```python
from build123d import *

# Parameters (mm, degrees)
SKETCH1_W                                            = 550
SKETCH1_H                                            = 360
BOSS_EXTRUDE1_DEPTH                                  = 5
SKETCH2_W                                            = 40
SKETCH2_H                                            = 15
CUT_EXTRUDE1_DEPTH                                   = 10
FILLET1_R                                            = 7.5
CHAMFER1_SIZE                                        = 50
SKETCH8_R                                            = 1.5
CUT_EXTRUDE5_DEPTH                                   = 10
CSK_FOR_M4_HEX_SOCKET_COUNTERSUNK_HEAD_S_D           = 4.5
CSK_FOR_M4_HEX_SOCKET_COUNTERSUNK_HEAD_S_CSINK_D     = 9.18
CSK_FOR_M4_HEX_SOCKET_COUNTERSUNK_HEAD_S_CSINK_ANGLE = 90
SKETCH10_R                                           = 2
CUT_EXTRUDE6_DEPTH                                   = 10
M5_TAPPED_HOLE1_D                                    = 4.2
M5_TAPPED_HOLE1_DEPTH                                = 12.4
M5_TAPPED_HOLE1_TIP                                  = 1.2618073
CUT_EXTRUDE8_REACH                                   = 330.71
SKETCH14_R                                           = 1.25
M3_TAPPED_HOLE1_D                                    = 2.5
M3_TAPPED_HOLE1_DEPTH                                = 7.5
M3_TAPPED_HOLE1_TIP                                  = 0.751075774
SKETCH16_R                                           = 1.5
CUT_EXTRUDE9_DEPTH                                   = 329.709598278
CSK_FOR_M4_HEX_SOCKET_COUNTERSUNK_HE_2_D             = 4.5
CSK_FOR_M4_HEX_SOCKET_COUNTERSUNK_HE_2_CSINK_D       = 9.18
CSK_FOR_M4_HEX_SOCKET_COUNTERSUNK_HE_2_CSINK_ANGLE   = 90


with BuildPart() as part:
    # Sketch1 → Boss-Extrude1 (new body)
    with BuildSketch(Plane(origin=(0, 0, 0), x_dir=(1, 0, 0), z_dir=(0, 1, 0))):
        Rectangle(SKETCH1_W, SKETCH1_H)
    extrude(amount=BOSS_EXTRUDE1_DEPTH)

    # Sketch2 → Cut-Extrude1 (cut)
    with BuildSketch(Plane(origin=(0, 5, 0), x_dir=(1, 0, 0), z_dir=(0, 1, 0))):
        with Locations((195, 0)):
            Rectangle(SKETCH2_W, SKETCH2_H)
        with Locations((-195, 0)):
            Rectangle(SKETCH2_W, SKETCH2_H)
    extrude(amount=-CUT_EXTRUDE1_DEPTH, mode=Mode.SUBTRACT)

    # Fillet1
    fillet1_edges = [part.edges().sort_by_distance(p)[0] for p in [
        (-175, 2.5, 7.5),
        (-175, 2.5, -7.5),
        (-215, 2.5, -7.5),
        (-215, 2.5, 7.5),
        (175, 2.5, 7.5),
        (175, 2.5, -7.5),
        (215, 2.5, -7.5),
        (215, 2.5, 7.5),
    ]]
    fillet(fillet1_edges, radius=FILLET1_R - 0.0001)  # a hair under: the kernel refuses the full size

    # Chamfer1
    chamfer1_edges = [part.edges().sort_by_distance(p)[0] for p in [
        (275, 2.5, 180),
        (-275, 2.5, 180),
        (-275, 2.5, -180),
        (275, 2.5, -180),
    ]]
    chamfer(chamfer1_edges, length=CHAMFER1_SIZE)

    # Sketch8 → Cut-Extrude5 (cut)
    with BuildSketch(Plane(origin=(0, 5, 0), x_dir=(1, 0, 0), z_dir=(0, 1, 0))):
        with Locations(Location((225, 5, 0), (0, 0, 270))):
            Circle(SKETCH8_R)
        with Locations(Location((165, 5, 0), (0, 0, 90))):
            Circle(SKETCH8_R)
        with Locations(Location((165, -5, 0), (0, 0, 270))):
            Circle(SKETCH8_R)
        with Locations(Location((225, -5, 0), (0, 0, 90))):
            Circle(SKETCH8_R)
        with Locations(Location((-225, -5, 0), (0, 0, 270))):
            Circle(SKETCH8_R)
        with Locations(Location((-165, -5, 0), (0, 0, 90))):
            Circle(SKETCH8_R)
        with Locations(Location((-165, 5, 0), (0, 0, 270))):
            Circle(SKETCH8_R)
        with Locations(Location((-225, 5, 0), (0, 0, 90))):
            Circle(SKETCH8_R)
    extrude(amount=-CUT_EXTRUDE5_DEPTH, mode=Mode.SUBTRACT)

    # CSK for M4 Hex Socket Countersunk Head S (through all)
    with Locations(Plane(origin=(-225, 5, -5), x_dir=(0, 0, 1), z_dir=(0, 1, 0))):
        with Locations((0, 0), (10, 0), (10, 60), (0, 60), (10, 390), (0, 390), (0, 450), (10, 450)):
            CounterSinkHole(CSK_FOR_M4_HEX_SOCKET_COUNTERSUNK_HEAD_S_D / 2, CSK_FOR_M4_HEX_SOCKET_COUNTERSUNK_HEAD_S_CSINK_D / 2, counter_sink_angle=CSK_FOR_M4_HEX_SOCKET_COUNTERSUNK_HEAD_S_CSINK_ANGLE)

    # Sketch10 → Cut-Extrude6 (cut)
    with BuildSketch(Plane(origin=(0, 5, 0), x_dir=(1, 0, 0), z_dir=(0, 1, 0))):
        with Locations(Location((237.5, 112, 0), (0, 0, 270))):
            Circle(SKETCH10_R)
        with Locations(Location((162.5, 112, 0), (0, 0, 90))):
            Circle(SKETCH10_R)
    extrude(amount=-CUT_EXTRUDE6_DEPTH, mode=Mode.SUBTRACT)

    # M5 Tapped Hole1
    with Locations(Plane(origin=(237.5, 5, -112), x_dir=(0, 0, 1), z_dir=(0, 1, 0))):
        with Locations((0, 0), (0, -75)):
            Hole(M5_TAPPED_HOLE1_D / 2, depth=M5_TAPPED_HOLE1_DEPTH)
            with Locations((0, 0, -(M5_TAPPED_HOLE1_DEPTH + M5_TAPPED_HOLE1_TIP / 2))):  # 118° drill point
                Cone(0, M5_TAPPED_HOLE1_D / 2, M5_TAPPED_HOLE1_TIP, mode=Mode.SUBTRACT)

    # Sketch14 → Cut-Extrude8 (cut, up to next)
    with BuildSketch(Plane(origin=(0, 5, 0), x_dir=(-1, 0, 0), z_dir=(0, 1, 0)), mode=Mode.PRIVATE) as cut_extrude8_sk1:
        with Locations(Location((-225, 25, 0), (0, 0, 90))):
            Circle(SKETCH14_R)
    cut_extrude8_tool1 = extrude(cut_extrude8_sk1.sketch, amount=-CUT_EXTRUDE8_REACH, mode=Mode.PRIVATE) & part.part
    # Sketch14 → Cut-Extrude8 (cut, up to next)
    with BuildSketch(Plane(origin=(0, 5, 0), x_dir=(-1, 0, 0), z_dir=(0, 1, 0)), mode=Mode.PRIVATE) as cut_extrude8_sk2:
        with Locations(Location((-225, -25, 0), (0, 0, 270))):
            Circle(SKETCH14_R)
    cut_extrude8_tool2 = extrude(cut_extrude8_sk2.sketch, amount=-CUT_EXTRUDE8_REACH, mode=Mode.PRIVATE) & part.part
    # Sketch14 → Cut-Extrude8 (cut, up to next)
    with BuildSketch(Plane(origin=(0, 5, 0), x_dir=(-1, 0, 0), z_dir=(0, 1, 0)), mode=Mode.PRIVATE) as cut_extrude8_sk3:
        with Locations(Location((-165, 25, 0), (0, 0, 270))):
            Circle(SKETCH14_R)
    cut_extrude8_tool3 = extrude(cut_extrude8_sk3.sketch, amount=-CUT_EXTRUDE8_REACH, mode=Mode.PRIVATE) & part.part
    # Sketch14 → Cut-Extrude8 (cut, up to next)
    with BuildSketch(Plane(origin=(0, 5, 0), x_dir=(-1, 0, 0), z_dir=(0, 1, 0)), mode=Mode.PRIVATE) as cut_extrude8_sk4:
        with Locations(Location((-165, -25, 0), (0, 0, 90))):
            Circle(SKETCH14_R)
    cut_extrude8_tool4 = extrude(cut_extrude8_sk4.sketch, amount=-CUT_EXTRUDE8_REACH, mode=Mode.PRIVATE) & part.part
    add(cut_extrude8_tool1.solids().sort_by_distance((225, 5, 25))[0], mode=Mode.SUBTRACT)
    add(cut_extrude8_tool2.solids().sort_by_distance((225, 5, -25))[0], mode=Mode.SUBTRACT)
    add(cut_extrude8_tool3.solids().sort_by_distance((165, 5, 25))[0], mode=Mode.SUBTRACT)
    add(cut_extrude8_tool4.solids().sort_by_distance((165, 5, -25))[0], mode=Mode.SUBTRACT)

    # M3 Tapped Hole1
    with Locations(Plane(origin=(225, 5, 25), x_dir=(0, 0, 1), z_dir=(0, 1, 0))):
        with Locations((0, 0), (0, -60), (-50, -60), (-50, 0)):
            Hole(M3_TAPPED_HOLE1_D / 2, depth=M3_TAPPED_HOLE1_DEPTH)
            with Locations((0, 0, -(M3_TAPPED_HOLE1_DEPTH + M3_TAPPED_HOLE1_TIP / 2))):  # 118° drill point
                Cone(0, M3_TAPPED_HOLE1_D / 2, M3_TAPPED_HOLE1_TIP, mode=Mode.SUBTRACT)

    # Sketch16 → Cut-Extrude9 (cut, through all)
    with BuildSketch(Plane(origin=(0, 5, 0), x_dir=(1, 0, 0), z_dir=(0, 1, 0))):
        with Locations(Location((38.6, 10.7, 0), (0, 0, 270))):
            Circle(SKETCH16_R)
        with Locations(Location((60, 10.7, 0), (0, 0, 270))):
            Circle(SKETCH16_R)
        with Locations(Location((38.6, -10.7, 0), (0, 0, 270))):
            Circle(SKETCH16_R)
        with Locations(Location((60, -10.7, 0), (0, 0, 270))):
            Circle(SKETCH16_R)
    extrude(amount=-CUT_EXTRUDE9_DEPTH, mode=Mode.SUBTRACT)

    # CSK for M4 Hex Socket Countersunk He 2 (through all)
    with Locations(Plane(origin=(60, 0, -10.7), x_dir=(0, 0, -1), z_dir=(0, -1, 0))):
        with Locations((0, 0), (0, -21.4), (-21.4, -21.4), (-21.4, 0)):
            CounterSinkHole(CSK_FOR_M4_HEX_SOCKET_COUNTERSUNK_HE_2_D / 2, CSK_FOR_M4_HEX_SOCKET_COUNTERSUNK_HE_2_CSINK_D / 2, counter_sink_angle=CSK_FOR_M4_HEX_SOCKET_COUNTERSUNK_HE_2_CSINK_ANGLE)


solid = part.part
```
Model file for the job. Use its own axes, mm. Coordinates: 2 decimals unless noted, no trailing zeros. Return JSON: item names as keys, results as strings. Group by question number.
1) Saw through at A-A, the plane y = 1.3. Count the separate pieces of the cut face and the enclosed holes in it, plus the area to 3 significant figures.
2) Flat gauge pins, fed straight in: P1, Ø2.5, axis at x = -225, z = -5, coming from the +Y side; P2, Ø7, axis at x = -225, z = 5, coming from the +Y side; P3, Ø5, axis at x = 38.6, z = -10.7, coming from the -Y side. Where does each tip first touch, or does it go through?
3) Probe line 1 (Z direction, x = 165, y = 1.9); line 2 (X direction, y = 1.6, z = 25); line 3 (Z direction, x = 39, y = 2.65). List the from-to ranges inside material, lowest first. Write a range as from..to.
Values found:
{
 "1": {"separate pieces": "1", "enclosed holes": "20", "area": "192,000 mm²"},
 "2": {"P1": "passes through", "P2": "stops at y = 3.91", "P3": "stops at y = 2.09"},
 "3": {"line 1": "z = -180..-26.25, -23.75..-7.25, -2.75..2.75, 7.25..23.75, 26.25..180", "line 2": "x = -275..163.75, 166.25..223.75, 226.25..275", "line 3": "z = -180..-12.91, -8.49..8.49, 12.91..180"}
}
